Here's how the part is built. I have some questions about the finished solid (model axes, mm). A direction names the side the tool comes from. Round coordinates to 2 decimals unless told otherwise and drop trailing zeros. Loops run counter-clockwise (first coordinate to the right, second up) from the corner with the lowest first, then second, coordinate; pieces in that order, holes last. Notation, with made-up numbers: M 47,70.5 L 104,70.5 A21 cw 104,89.5 Z; hole C 63,33 d7. An arc over 180 degrees is marked long. Use a Markdown table: item, result.
from build123d import *

# Parameters (mm, degrees)
SKETCH2_R           = 14.2875
BOSS_EXTRUDE1_DEPTH = 3.175


with BuildPart() as part:
    # Sketch2 → Boss-Extrude1 (new body)
    with BuildSketch(Plane.XY):
        with BuildLine():
            Line((-252.633177849, 218.001908783), (-176.433177849, 68.837869886))
            ThreePointArc((-176.433177849, 68.837869886), (-174.97190788, 66.322103076), (-173.24831347, 63.978256905))
            Line((-173.24831347, 63.978256905), (-106.57331347, -17.136889499))
            ThreePointArc((-106.57331347, -17.136889499), (-97.254166295, -24.400890984), (-85.725, -26.9875))
            Line((-85.725, -26.9875), (85.725, -26.9875))
            ThreePointArc((85.725, -26.9875), (97.254166295, -24.400890984), (106.57331347, -17.136889499))
            Line((106.57331347, -17.136889499), (173.24831347, 63.978256905))
            ThreePointArc((173.24831347, 63.978256905), (174.97190788, 66.322103076), (176.433177849, 68.837869886))
            Line((176.433177849, 68.837869886), (252.633177849, 218.001908783))
            ThreePointArc((252.633177849, 218.001908783), (240.877276518, 254.31236315), (204.566822151, 242.556461819))
            Line((204.566822151, 242.556461819), (129.696163279, 95.994652474))
            Line((129.696163279, 95.994652474), (72.973687944, 26.9875))
            Line((72.973687944, 26.9875), (-72.973687944, 26.9875))
            Line((-72.973687944, 26.9875), (-129.696163279, 95.994652474))
            Line((-129.696163279, 95.994652474), (-204.566822151, 242.556461819))
            ThreePointArc((-204.566822151, 242.556461819), (-240.877276518, 254.31236315), (-252.633177849, 218.001908783))
        make_face()
        with Locations((-228.6, 230.279185301)):
            Circle(SKETCH2_R, mode=Mode.SUBTRACT)
        with Locations((-152.4, 81.115146404)):
            Circle(SKETCH2_R, mode=Mode.SUBTRACT)
        with Locations((-85.725, 0)):
            Circle(SKETCH2_R, mode=Mode.SUBTRACT)
        with Locations((85.725, 0)):
            Circle(SKETCH2_R, mode=Mode.SUBTRACT)
        with Locations((152.4, 81.115146404)):
            Circle(SKETCH2_R, mode=Mode.SUBTRACT)
        with Locations((228.6, 230.279185301)):
            Circle(SKETCH2_R, mode=Mode.SUBTRACT)
    extrude(amount=BOSS_EXTRUDE1_DEPTH)


solid = part.part
1. For pin 1 Ø1 at (y, z) = (137.5, 0.5) entering from +X; pin 2 Ø1.5 at (y, z) = (78.5, 2.5) entering from +X; pin 3 Ø17 at (x, y) = (-152.4, 81.12) entering from -Z, each with a flat end and sliding along its axis, tell me the tip position at first contact or that it passes through.
Answer sheet:
| item | result |
|---|---|
| pin 1 | x = 211.76 |
| pin 2 | x = 181.75 |
| pin 3 | through |
2. We'd pull the mould along X, two halves only. Please class faces 3 (the face through (-215.067, 144.464, 1.565)), 4 (the face through (-1, 21, 0)), 5 (the face through (-100, 0.6, 1.6)): +X half, -X half, draft (parallel to the pull), parting line (faces both ways), or undercut.
Answer sheet:
| item | result |
|---|---|
| face 3 | -X half |
| face 4 | draft |
| face 5 | undercut |
3. I need wall thicknesses on probe 1 along X at (y, z) = (241, 2.7); probe 2 along Y at (x, z) = (60.5, 1.8); probe 3 along X at (y, z) = (234.5, 0.2). Which ranges of each line are inside material? Lowest first, please. Write a range as from..to.
Answer sheet:
| item | result |
|---|---|
| probe 1 | -253.37..-238.04, -219.16..-203.77, 203.77..219.16, 238.04..253.37 |
| probe 2 | -26.99..26.99 |
| probe 3 | -255.26..-242.25, -214.95..-200.45, 200.45..214.95, 242.25..255.26 |
4. Imagine slicing it at B-B, the plane y = 90. Write out the boundary of the cut face in (x, z) (3 decimals).
Answer sheet:
| item | result |
|---|---|
| outline | M -187.244,0 L -163.589,0 L -163.589,3.175 L -187.244,3.175 Z; M -141.211,0 L -124.769,0 L -124.769,3.175 L -141.211,3.175 Z; M 124.769,0 L 141.211,0 L 141.211,3.175 L 124.769,3.175 Z; M 163.589,0 L 187.244,0 L 187.244,3.175 L 163.589,3.175 Z |
5. Imagine slicing it at D-D, the plane z = 0.7. Write out the boundary of the cut face in (x, y) (1 decimal).
Answer sheet:
| item | result |
|---|---|
| outline | M -252.6,218 L -176.4,68.8 A27 ccw -173.2,64 L -106.6,-17.1 A27 ccw -85.7,-27 L 85.7,-27 A27 ccw 106.6,-17.1 L 173.2,64 A27 ccw 176.4,68.8 L 252.6,218 A27 ccw 204.6,242.6 L 129.7,96 L 73,27 L -73,27 L -129.7,96 L -204.6,242.6 A27 ccw Z; hole C -228.6,230.3 d28.6; hole C -152.4,81.1 d28.6; hole C -85.7,0 d28.6; hole C 85.7,0 d28.6; hole C 152.4,81.1 d28.6; hole C 228.6,230.3 d28.6 |
6. Which directions (+Z, -Z, +X, -X, +Y, -Y) give clear straight access to the entire face, cutting with the end or side of a thin tool? Please do faces 1 (the face through (-100.94, 61.01, 1.57)), 2 (the face through (214, 142.38, 1.57)).
Answer sheet:
| item | result |
|---|---|
| face 1 | +Z, -Z, +Y |
| face 2 | +Z, -Z, +X, -Y |
7. Imagine slicing it at A-A, the plane x = -228.6. Write out the boundary of the cut face in (y, z) (3 decimals), then the cut area to 3 significant figures.
Answer sheet:
| item | result |
|---|---|
| outline | M 170.956,0 L 215.992,0 L 215.992,3.175 L 170.956,3.175 Z; M 244.567,0 L 257.267,0 L 257.267,3.175 L 244.567,3.175 Z |
| area | 183 mm2 |
8. Imagine slicing it at C-C, the plane y = 0. Write out the boundary of the cut face in (x, z) (1 decimal), then the cut area to 3 significant figures.
Answer sheet:
| item | result |
|---|---|
| outline | M -120.7,0 L -100,0 L -100,3.2 L -120.7,3.2 Z; M -71.4,0 L 71.4,0 L 71.4,3.2 L -71.4,3.2 Z; M 100,0 L 120.7,0 L 120.7,3.2 L 100,3.2 Z |
| area | 585 mm2 |
